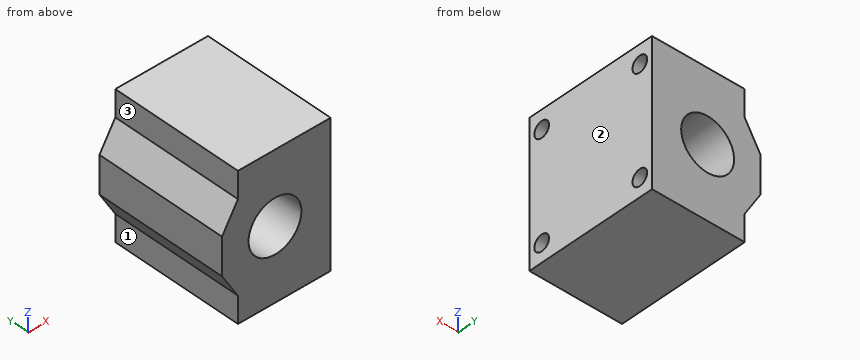
```python
from build123d import *

# Parameters (mm, degrees)
F1_DEPTH = 25
F2_R     = 10
F3_DEPTH = 50
F4_R     = 3
F5_DEPTH = 12


with BuildPart() as f1:
    # F0 (on Front) → F1 (new body, symmetric)
    with BuildSketch(Plane.XZ):
        Polygon((20.5, -27), (20.5, 27), (-14.5, 27), (-14.5, 17), (-20.5, 7), (-20.5, -7), (-14.5, -17), (-14.5, -27), align=None)
    extrude(amount=F1_DEPTH, both=True)

    # F2 (on face) → F3 (cut)
    with BuildSketch(Plane.XZ.offset(25)):
        with Locations((-0.5, 0)):
            Circle(F2_R)
    extrude(amount=-F3_DEPTH, mode=Mode.SUBTRACT)

    # F4 (on face) → F5 (cut)
    with BuildSketch(Plane.YZ.offset(20.5)):
        with Locations((-20, 20)):
            Circle(F4_R)
        with Locations((20, 20)):
            Circle(F4_R)
        with Locations((20, -20)):
            Circle(F4_R)
        with Locations((-20, -20)):
            Circle(F4_R)
    extrude(amount=-F5_DEPTH, mode=Mode.SUBTRACT)


solid = f1.part
```
The listing builds one solid part. Answer for the finished solid, in the listing's coordinates (mm). Face numbers are marked on the shaded views. A direction names the side the tool comes from. Round coordinates to 2 decimals unless told otherwise and drop trailing zeros. Order: outer loops, then holes, each group sorted by start corner. A loop starts at its lowest first (then second) coordinate and runs counter-clockwise, first axis right, second up. Notation, with made-up numbers: (17, 18) - (48, 18) arc R16 ccw to (48, 30) - close; hole circle Ø1 at (83, -18.5). An arc over 180 degrees is marked (long way). Put each result on its own line as item: value. Start each with the question number.
(1) Find section A-A (z = 0). Give the vertices of the cut face in (x, y), plus the area to 3 significant figures.
(2) Find section D-D (x = 14). Give the vertices of the cut face in (y, z).
(3) Given P1, Ø3, axis at y = 21.5, z = -21, coming from the +X side; P2, Ø1.5, axis at y = 15.5, z = 11.5, coming from the -X side; P3, Ø4, axis at y = -4.5, z = -21.5, coming from the -X side; P4, Ø5.5, axis at y = -20, z = 20, coming from the +X side, each flat-ended and moving along its own axis, determine where each tip first touches the part or whether it passes through.
(4) Find section B-B (y = 4). Give the vertices of the cut face in (x, z).
(5) For the marked faces 1, 2 and 3, determine the directions among +Z, -Z, +X, -X, +Y, -Y from which every point of the face is accessible in a straight line to the end or side of a thin tool.
(6) Find section C-C (x = -0.5). Give the vertices of the cut face in (y, z).
(7) Straight lines are drawn through the part: probe 1 along Z at (x, y) = (15.75, -20); probe 2 along Z at (x, y) = (-1, -11); probe 3 along X at (y, z) = (22, 18). For each, find the intervals that lie inside material, in ascending order. Write a range as from..to.
Reply:
1. outline: (-20.5, -25) - (-10.5, -25) - (-10.5, 25) - (-20.5, 25) - close; (9.5, -25) - (20.5, -25) - (20.5, 25) - (9.5, 25) - close
1. area: 1,050 mm^2
2. outline: (-25, -27) - (25, -27) - (25, 27) - (-25, 27) - close; hole circle Ø6 at (-20, -20); hole circle Ø6 at (-20, 20); hole circle Ø6 at (20, -20); hole circle Ø6 at (20, 20)
3. P1: x = 20.5
3. P2: x = -18.25
3. P3: x = -14.5
3. P4: x = 8.5
4. outline: (-20.5, -7) - (-14.5, -17) - (-14.5, -27) - (20.5, -27) - (20.5, 27) - (-14.5, 27) - (-14.5, 17) - (-20.5, 7) - close; hole circle Ø20 at (-0.5, 0)
5. face 1: -Z, -X, +Y, -Y
5. face 2: +Z, -Z, +X, +Y, -Y
5. face 3: +Z, -X, +Y, -Y
6. outline: (-25, -27) - (25, -27) - (25, -10) - (-25, -10) - close; (-25, 10) - (25, 10) - (25, 27) - (-25, 27) - close
7. probe 1: -27..-23, -17..17, 23..27
7. probe 2: -27..-9.99, 9.99..27
7. probe 3: -14.5..8.5
